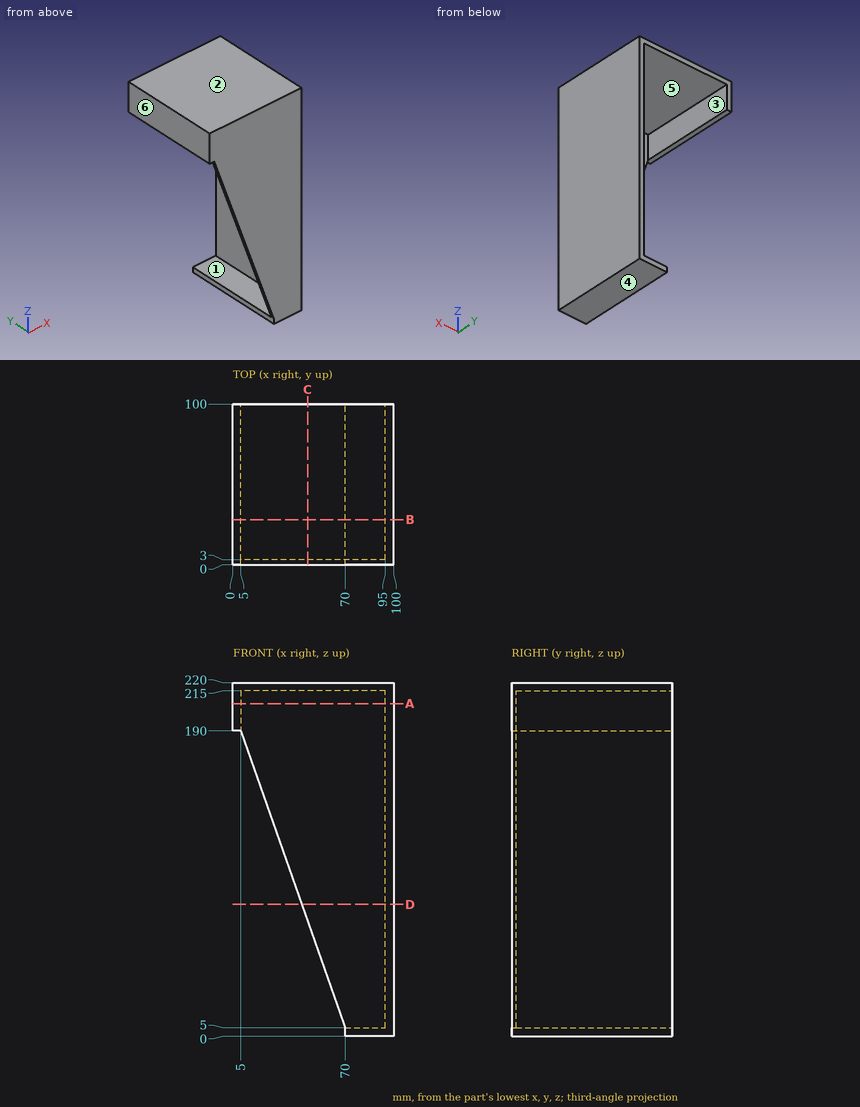
Print and shaded views of the part. All mm, measured from the part's lowest x, y and z. A direction names the side the tool comes from. Coordinates: 2 decimals unless noted, no trailing zeros. Write each loop counter-clockwise with the first axis right and the second up, starting at its lowest first coordinate (ties: lowest second). Pieces come first, ordered by that corner, then holes. Notation, with made-up numbers: (64.5, 61) -> (96.5, 61) arc R29 cw to (96.5, 100) -> close; hole circle Ø7 at (-23, 69). An arc over 180 degrees is marked (long way). Use CSV: the item, a comma, the result in double quotes. Start each with the question number.
Q1. Cut at B-B, the plane y = 28. List the corners of the cut face in (x, z), then the cut area to 4 significant figures.
Q2. Flat gauge pins, fed straight in: pin 1 Ø3 at (x, z) = (84.5, 180) entering from -Y; pin 2 Ø6 at (x, y) = (11, 72.5) entering from -Z; pin 3 Ø6 at (x, z) = (58, 50) entering from +Y; pin 4 Ø4 at (y, z) = (57, 2) entering from -X. Where does each tip first touch, or does it go through?
Q3. 3-axis set-ups, long thin cutter, end or side, ignore diameter. For the marked faces 1, 2 and 3: which of +Z, -Z, +X, -X, +Y, -Y reach the whole face in a straight line?
Q4. Cut at D-D, the plane z = 82. List the corners of the cut face in (x, y), then the cut area to 3 significant figures.
Q5. Cut at A-A, the plane z = 207. List the corners of the cut face in (x, y), then the cut area to 3 significant figures.
Q6. Cut at C-C, the plane x = 46.5. List the corners of the cut face in (y, z).
Q7. Pull direction X, two halves, no side cores. Call the marked faces 4, 5 and 6: released by +X, released by -X, zero draft, split by the parting line, or undercut.
Q8. Drill centre lines: probe 1 along X at (y, z) = (71, 206.5); probe 2 along Z at (x, y) = (93, 54); probe 3 along X at (y, z) = (84, 49). Where is each one in solid material? Low to high.
Checked values:
1,outline,"(0, 190) -> (5, 190) -> (5, 215) -> (95, 215) -> (95, 5) -> (70, 5) -> (70, 0) -> (100, 0) -> (100, 220) -> (0, 220) -> close"
1,area,"1,825 mm²"
2,pin 1,"stops at y = 0"
2,pin 2,"stops at z = 215"
2,pin 3,"stops at y = 3"
2,pin 4,"stops at x = 70"
3,face 1,"-X, +Y"
3,face 2,"+Z, +X, -X, +Y, -Y"
3,face 3,"-Z, +Y"
4,outline,"(42.95, 0) -> (100, 0) -> (100, 100) -> (95, 100) -> (95, 3) -> (42.95, 3) -> close"
4,area,"656 mm²"
5,outline,"(0, 0) -> (100, 0) -> (100, 100) -> (95, 100) -> (95, 3) -> (5, 3) -> (5, 100) -> (0, 100) -> close"
5,area,"1,270 mm²"
6,outline,"(0, 71.88) -> (3, 71.88) -> (3, 215) -> (100, 215) -> (100, 220) -> (0, 220) -> close"
7,face 4,"zero draft"
7,face 5,"undercut"
7,face 6,"released by -X"
8,probe 1,"x = 0 to 5, 95 to 100"
8,probe 2,"z = 0 to 5, 215 to 220"
8,probe 3,"x = 95 to 100"
